The figure shows three views and two pictorial views of one solid part (mm, origin at its lowest corner). Answer the questions. A direction names the side the tool comes from. Give positions to 0.01 mm unless a question says otherwise; leave off trailing zeros. Order: outer loops, then holes, each group sorted by start corner. A loop starts at its lowest first (then second) coordinate and runs counter-clockwise, first axis right, second up. Notation, with made-up numbers: (84.5, 26) - (106.5, 26) arc R16 cw to (106.5, 30) - close; hole circle Ø3 at (59.5, 19). An arc over 180 degrees is marked (long way). Return JSON: item names as keys, results as strings. Group by question number.
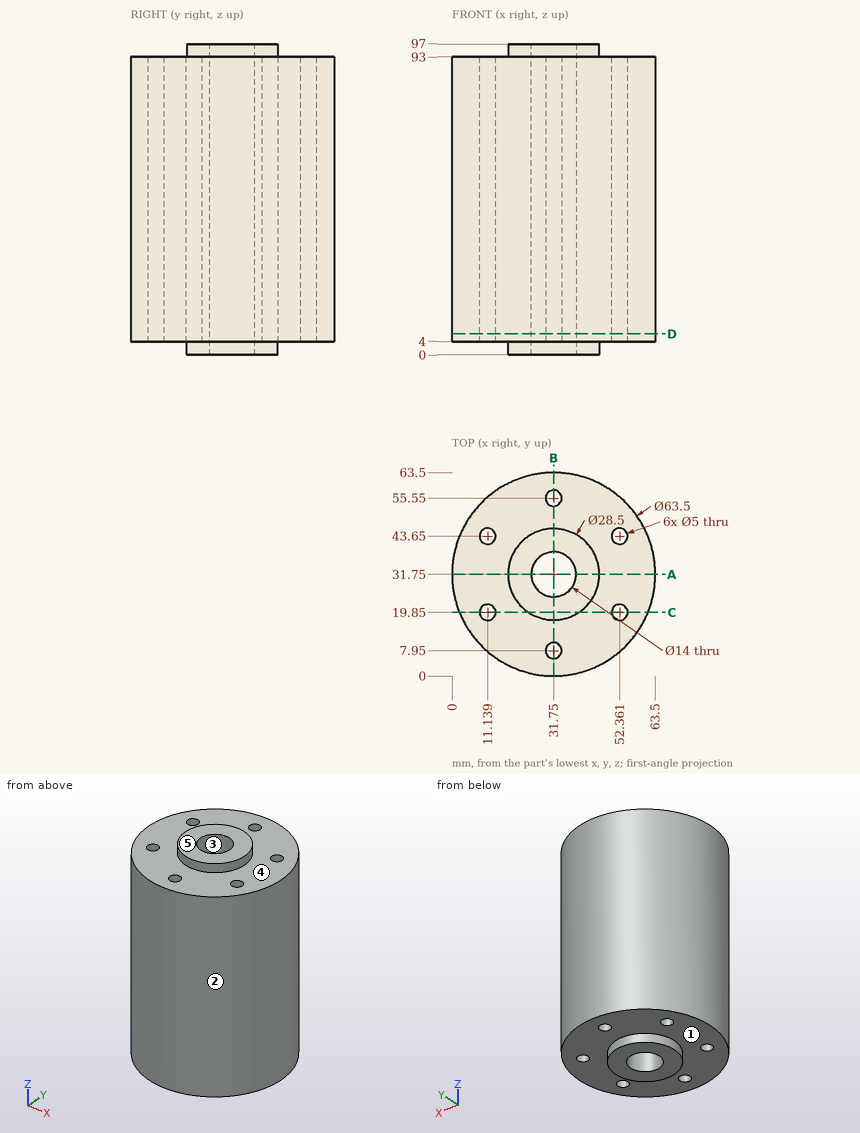
1. A tool of negligible diameter and unlimited length cuts with its end or side. For the marked faces 4 and 5, from which of +Z, -Z, +X, -X, +Y, -Y can it reach the whole face along a straight path? Write none if from no direction.
2. The part is cut by section C-C (y = 19.85). Give the vertices of the cut face in (x, z) (1 decimal).
3. Consider probe 1 along Y at (x, z) = (31.75, 31); probe 2 along Y at (x, z) = (52, 60.5) (1 decimal); probe 3 along Y at (x, z) = (31, 39) (1 decimal). Determine where each line is inside the solid, lowest interval first. Write a range as from..to.
4. Each of these flat-tipped pins is pushed along its axis until it touches: pin 1 (4 mm diameter, centred on x = 24, z = 19, fed in from +Y) (1 decimal); pin 2 (3 mm diameter, centred on x = 31.75, y = 7.95, fed in from +Z); pin 3 (6.5 mm diameter, centred on x = 11.14, y = 43.65, fed in from +Z); pin 4 (12 mm diameter, centred on x = 15.5, y = 53.5, fed in from -Z). Where does it stop, or does it pass through?
5. The part is cut by section A-A (y = 31.75). Give the vertices of the cut face in (x, z), and give its area (3 significant figures).
6. Determine the mould class of the marked faces 1, 2 and 3 for opening direction Y: released by +Y, released by -Y, zero draft, split by the parting line, or undercut.
7. The part is cut by section D-D (z = 6.5). State how many separate pieces and enclosed holes the cut face has, and give its area (4 significant figures).
8. The part is cut by section B-B (x = 31.75). Give the vertices of the cut face in (y, z), and give its area (3 significant figures).
Answers:
{
 "1": {"face 4": "+Z", "face 5": "+Z, +X, -X, +Y, -Y"},
 "2": {"outline": "(2.3, 4) - (8.6, 4) - (8.6, 93) - (2.3, 93) - close; (13.6, 4) - (23.9, 4) - (23.9, 0) - (39.6, 0) - (39.6, 4) - (49.9, 4) - (49.9, 93) - (39.6, 93) - (39.6, 97) - (23.9, 97) - (23.9, 93) - (13.6, 93) - close; (54.9, 4) - (61.2, 4) - (61.2, 93) - (54.9, 93) - close"},
 "3": {"probe 1": "y = 0..5.45, 10.45..24.75, 38.75..53.05, 58.05..63.5", "probe 2": "y = 7.3..17.4, 22.3..41.2, 46.1..56.2", "probe 3": "y = 0..5.6, 10.3..24.8, 38.7..53.2, 57.9..63.5"},
 "4": {"pin 1": "stops at y = 63", "pin 2": "passes through", "pin 3": "stops at z = 93", "pin 4": "stops at z = 4"},
 "5": {"outline": "(0, 4) - (17.5, 4) - (17.5, 0) - (24.75, 0) - (24.75, 97) - (17.5, 97) - (17.5, 93) - (0, 93) - close; (38.75, 0) - (46, 0) - (46, 4) - (63.5, 4) - (63.5, 93) - (46, 93) - (46, 97) - (38.75, 97) - close", "area": "4,520 mm^2"},
 "6": {"face 1": "zero draft", "face 2": "split by the parting line", "face 3": "undercut"},
 "7": {"separate pieces": "1", "enclosed holes": "7", "area": "2,895 mm^2"},
 "8": {"outline": "(0, 4) - (5.45, 4) - (5.45, 93) - (0, 93) - close; (10.45, 4) - (17.5, 4) - (17.5, 0) - (24.75, 0) - (24.75, 97) - (17.5, 97) - (17.5, 93) - (10.45, 93) - close; (38.75, 0) - (46, 0) - (46, 4) - (53.05, 4) - (53.05, 93) - (46, 93) - (46, 97) - (38.75, 97) - close; (58.05, 4) - (63.5, 4) - (63.5, 93) - (58.05, 93) - close", "area": "3,630 mm^2"}
}
